from build123d import *

# Parameters (mm, degrees)
SKETCH1_R           = 300
BOSS_EXTRUDE1_DEPTH = 300
SKETCH2_R           = 30
BOSS_EXTRUDE2_DEPTH = 200
SKETCH3_R           = 300
BOSS_EXTRUDE3_DEPTH = 100


with BuildPart() as part:
    # Sketch1 → Boss-Extrude1 (new body)
    with BuildSketch(Plane(origin=(0, 0, 0), x_dir=(1, 0, 0), z_dir=(0, 1, 0))):
        Circle(SKETCH1_R)
    extrude(amount=BOSS_EXTRUDE1_DEPTH)

    # Sketch2 → Boss-Extrude2 (add)
    with BuildSketch(Plane(origin=(0, 300, 0), x_dir=(1, 0, 0), z_dir=(0, 1, 0))):
        with Locations((0, 250)):
            Circle(SKETCH2_R)
        with Locations((0, -250)):
            Circle(SKETCH2_R)
    extrude(amount=BOSS_EXTRUDE2_DEPTH)

    # Sketch3 → Boss-Extrude3 (add)
    with BuildSketch(Plane(origin=(0, 500, 0), x_dir=(1, 0, 0), z_dir=(0, 1, 0))):
        Circle(SKETCH3_R)
    extrude(amount=BOSS_EXTRUDE3_DEPTH)


solid = part.part
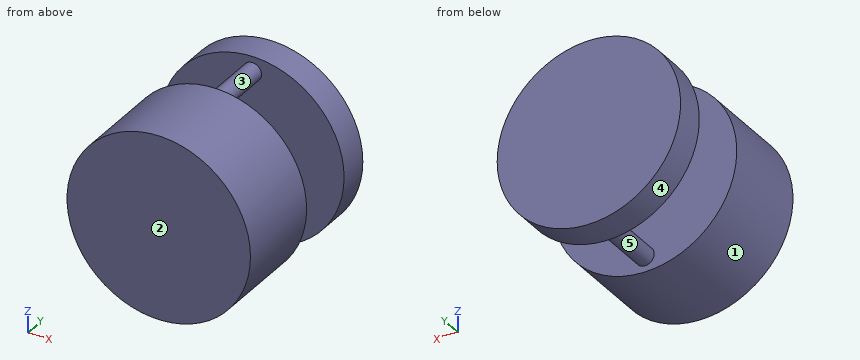
The listing builds one solid part. Answer for the finished solid, in the listing's coordinates (mm). Face numbers are marked on the shaded views. A direction names the side the tool comes from. Coordinates: 2 decimals unless noted, no trailing zeros. Write each loop counter-clockwise with the first axis right and the second up, starting at its lowest first coordinate (ties: lowest second). Pieces come first, ordered by that corner, then holes. Notation, with made-up numbers: M 57.25,7.25 L 106.25,7.25 A15 ccw 106.25,34.25 Z; hole C -31,40 d7. An arc over 180 degrees is marked long. Put each result on its own line as item: value. Start each with the question number.
1. For a pull along Z with two mould halves and no side action, classify the marked faces 1, 2 and 3 as pulls with the +Z half, pulls with the -Z half, needs draft (parallel to the pull), parting line crosses it, or undercut.
2. Consider line 1 (Y direction, x = 237.5, z = 180); line 2 (X direction, y = 279, z = 198); line 3 (Z direction, x = -91, y = 508). Determine where each line is inside the solid, lowest interval first. Write a range as from..to.
3. A cutting plane is placed at D-D on y = 350. Write down the section's boundary in (x, z).
4. A cutting plane is placed at B-B on z = 0. Write down the section's boundary in (x, y).
5. A cutting plane is placed at C-C on x = 214. Write down the section's boundary in (y, z), then the cut area to 3 significant figures.
6. A cutting plane is placed at A-A on x = 0. Write down the section's boundary in (y, z), then the cut area to 3 significant figures.
7. Flat-ended cylindrical pins translate along their axes: P1, Ø6, axis at y = 109.5, z = -199, coming from the -X side; P2, Ø1.5, axis at x = 22, y = 323, coming from the +Z side; P3, Ø4, axis at y = 523, z = 133.5, coming from the -X side. Find the tip coordinate at first contact, or state that the pin passes through.
8. Which of the six approach directions +Z, -Z, +X, -X, +Y, -Y give full straight-line access (tool end or side, diameter ignored) to the marked faces 4 and 5?
Resolved:
1. face 1: parting line crosses it
1. face 2: needs draft
1. face 3: undercut
2. line 1: y = 0..300, 500..600
2. line 2: x = -225.38..225.38
2. line 3: z = -285.87..285.87
3. outline: C 0,-250 d60; C 0,250 d60
4. outline: M -300,0 L 300,0 L 300,300 L -300,300 Z; M -300,500 L 300,500 L 300,600 L -300,600 Z
5. outline: M 0,-210.25 L 300,-210.25 L 300,210.25 L 0,210.25 Z; M 500,-210.25 L 600,-210.25 L 600,210.25 L 500,210.25 Z
5. area: 168,000 mm2
6. outline: M 0,-300 L 300,-300 L 300,-280 L 500,-280 L 500,-300 L 600,-300 L 600,300 L 500,300 L 500,280 L 300,280 L 300,300 L 0,300 Z; hole M 300,-220 L 500,-220 L 500,220 L 300,220 Z
6. area: 264,000 mm2
7. P1: stops at x = -227.12
7. P2: stops at z = 271.18
7. P3: stops at x = -269.64
8. face 4: +Y, -Y
8. face 5: none
